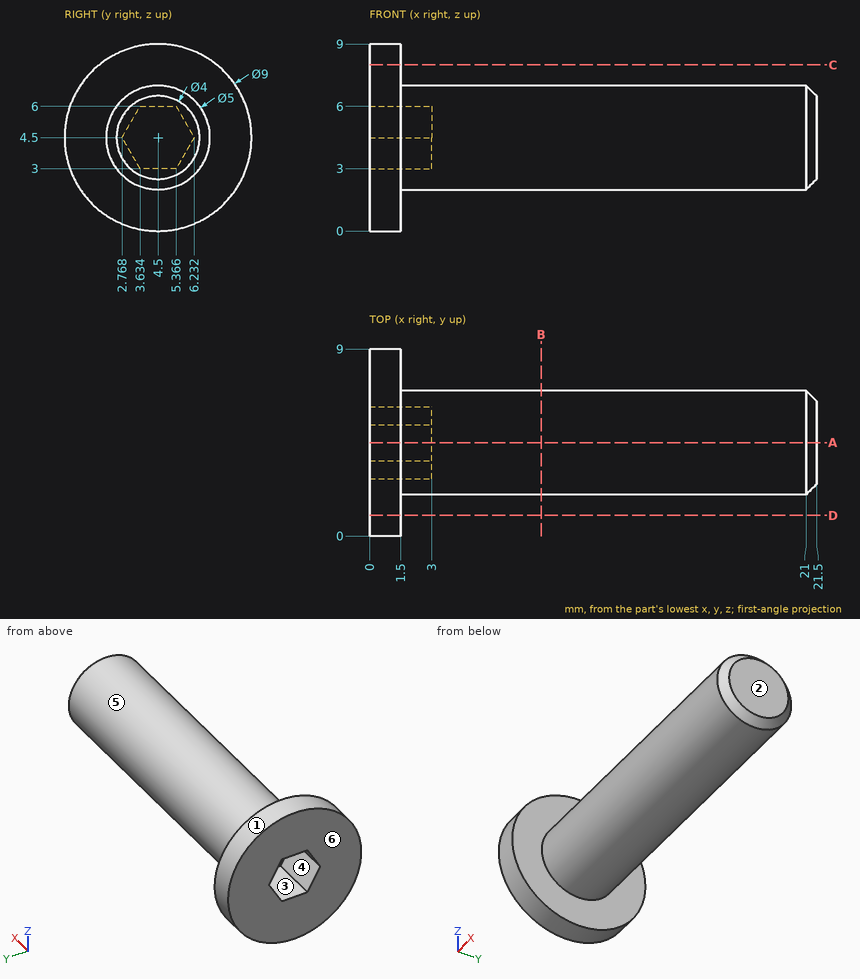
Design review of the part shown in the three views and the two pictorial views. Dimensions are in mm from the part's minimum x, y and z. A direction names the side the tool comes from. Round coordinates to 2 decimals unless told otherwise and drop trailing zeros. Write each loop counter-clockwise with the first axis right and the second up, starting at its lowest first coordinate (ties: lowest second). Pieces come first, ordered by that corner, then holes. Notation, with made-up numbers: (13.25, -4.5) -> (53.25, -4.5) arc R27 cw to (53.25, 23.5) -> close; hole circle Ø4 at (62, 35.5). An arc over 180 degrees is marked (long way). One line per question, with ' | ' between items. Start each with the question number.
1) Mouldability with a two-part tool opening along Z and no side actions: class the marked faces 1, 2, 3 and 4 as +Z half, -Z half, draft (parallel to the pull), parting line (faces both ways), or undercut.
2) Machinability: for the marked faces 5 and 6, which of the approach directions +Z, -Z, +X, -X, +Y, -Y give a long, thin tool a straight path to every point of the face, cutting with its end or side? Answer none if there is none.
3) Add section C-C (z = 8). Write out the cut boundary in (x, y).
4) Add section A-A (y = 4.5). Write out the cut boundary in (x, z).
5) Wall thickness on line 1 along X through (y, z) = (7, 5); line 2 along X through (y, z) = (3.75, 5.25); line 3 along Z through (x, y) = (2, 4.25): over which ranges is each line inside the solid? List them lowest first.
6) Add section B-B (x = 8.25). Write out the cut boundary in (y, z), and give its area (3 significant figures).
7) For pin 1 Ø1.5 at (x, y) = (7.5, 3) entering from +Z; pin 2 Ø2 at (x, y) = (3, 6.5) entering from +Z; pin 3 Ø2 at (y, z) = (7, 7.5) entering from +X, all flat-tipped, find the tip position at first contact; note any pin that passes through.
Reported:
1) face 1: parting line | face 2: draft | face 3: undercut | face 4: undercut
2) face 5: +X | face 6: +Z, -Z, -X, +Y, -Y
3) outline: (0, 1.67) -> (1.5, 1.67) -> (1.5, 7.33) -> (0, 7.33) -> close
4) outline: (0, 0) -> (1.5, 0) -> (1.5, 2) -> (21, 2) -> (21.5, 2.5) -> (21.5, 6.5) -> (21, 7) -> (1.5, 7) -> (1.5, 9) -> (0, 9) -> (0, 6) -> (3, 6) -> (3, 3) -> (0, 3) -> close
5) line 1: x = 0 to 1.5 | line 2: x = 3 to 21.5 | line 3: z = 2.01 to 3, 6 to 6.99
6) outline: circle Ø5 at (4.5, 4.5) | area: 19.6 mm²
7) pin 1: stops at z = 6.88 | pin 2: stops at z = 6.79 | pin 3: stops at x = 1.5
